```python
from build123d import *

# Parameters (mm, degrees)
F1_DEPTH = 4
F2_R     = 10
F3_R     = 2
F4_W     = 17
F4_H     = 8
F5_DEPTH = 3


with BuildPart() as f1:
    # F0 (on Top) → F1 (new body, symmetric)
    with BuildSketch(Plane.XY):
        with BuildLine():
            Line((31.1703724303, -13.5), (34.3061052263, 0))
            Line((34.3061052263, 0), (17.3061052263, 0))
            ThreePointArc((17.3061052263, 0), (22.6203428996, -9.4465185643), (19.5969211067, -19.8550129652))
            ThreePointArc((19.5969211067, -19.8550129652), (19.9679460836, -23.371024977), (23.4839580953, -23))
            Line((23.4839580953, -23), (31.1703724303, -13.5))
        make_face()
    extrude(amount=F1_DEPTH, both=True)

    # F2
    f2_edges = [f1.edges().sort_by_distance(p)[0] for p in [
        (31.170372, -13.5, 0),
    ]]
    fillet(f2_edges, radius=F2_R)

    # F3
    f3_edges = [f1.edges().sort_by_distance(p)[0] for p in [
        (32.998368, -5.630086, 4),
        (30.935867, -13.38549, 4),
        (26.603989, -19.143807, 4),
        (19.967946, -23.371025, 4),
        (22.620343, -9.446519, 4),
        (22.620343, -9.446519, -4),
        (19.967946, -23.371025, -4),
        (26.603989, -19.143807, -4),
        (30.935867, -13.38549, -4),
        (32.998368, -5.630086, -4),
    ]]
    fillet(f3_edges, radius=F3_R)

    # F4 (on face) → F5 (join)
    with BuildSketch(Plane(origin=(0, 0, 0), x_dir=(-1, 0, 0), z_dir=(0, 1, 0))):
        with Locations((-25.8061052263, 0)):
            Rectangle(F4_W, F4_H)
    extrude(amount=F5_DEPTH)


solid = f1.part
```
Check sheet for the modelled part. Datum: model origin and axes. Units: mm. A direction names the side the tool comes from. Give positions to 0.01 mm unless a question says otherwise; leave off trailing zeros. Order: outer loops, then holes, each group sorted by start corner. A loop starts at its lowest first (then second) coordinate and runs counter-clockwise, first axis right, second up. Notation, with made-up numbers: M -31.5,-29.75 L -16.5,-29.75 A37 cw -16.5,6.25 Z; hole C 48.25,67 d3. An arc over 180 degrees is marked long. Answer in a Markdown table with one row per item. Add a question column.
Q1. Thickness scan on L1, parallel to Y at x = 21, z = 2.25; L2, parallel to X at y = -5.5, z = -1.75; L3, parallel to Y at x = 26.5, z = -0.5. Record the ranges inside material, lowest first.
Q2. Release check for a two-part mould opening along Y. For faces 1 (the cylindrical face through (19.93, -23.34, 0.03)), 2 (the flat face through (26, -4, 4)), 3 (the cylindrical face through (30.95, -13.36, -0.03)) record: released by +Y, released by -Y, zero draft, split by the parting line, or undercut.
Q3. Access from +Z, -Z, +X, -X, +Y, -Y to the whole of each face (thin tool, end or side, straight path). Record for faces 4 (the flat face through (33.9, 0, 3.5)), 5 (the flat face through (18, 0, 3.6)), 6 (the flat face through (18, 0, -3.6)), 7 (the cylindrical face through (22.6, -9.29, 0.03)), 8 (the flat face through (33.9, 0, -3.5)).
Q4. Gauge pin test, flat ends, axial feed: pin 1 Ø2 at (y, z) = (-14, 1.5) entering from +X; pin 2 Ø10 at (x, y) = (32, -7.5) entering from -Z; pin 3 Ø1.5 at (y, z) = (-12, -3) entering from +X; pin 4 Ø1 at (x, z) = (19, -3) entering from -Y. Record the tip position at first contact, or that the pin passes through.
Q5. Sectioned sample at A-A, the plane z = -1. Record the boundary of the cut face in (x, y), and give its area (3 significant figures).
Verdict:
| question | item | result |
|---|---|---|
| 1 | L1 | -23.85 to -17.79, -4.31 to 3 |
| 1 | L2 | 21.56 to 33.03 |
| 1 | L3 | -19.27 to 3 |
| 2 | face 1 | undercut |
| 2 | face 2 | zero draft |
| 2 | face 3 | released by -Y |
| 3 | face 4 | +Z, +X, -Y |
| 3 | face 5 | +Z, -X, -Y |
| 3 | face 6 | -Z, -X, -Y |
| 3 | face 7 | +Z, -Z, -X |
| 3 | face 8 | -Z, +X, -Y |
| 4 | pin 1 | x = 31.11 |
| 4 | pin 2 | z = -4 |
| 4 | pin 3 | x = 31.58 |
| 4 | pin 4 | y = -22.48 |
| 5 | outline | M 17.31,0 A14 cw 19.6,-19.86 A2.5 ccw 23.48,-23 L 29.72,-15.29 A10 ccw 31.69,-11.26 L 34.31,0 L 34.31,3 L 17.31,3 Z |
| 5 | area | 270 mm² |
